For this review, use the dimensioned drawing (mm, ordinates from the lowest corner) and the shaded views. Give positions to 0.01 mm unless a question says otherwise; leave off trailing zeros. Order: outer loops, then holes, each group sorted by start corner. A loop starts at its lowest first (then second) coordinate and runs counter-clockwise, first axis right, second up. Notation, with made-up numbers: M 27.25,75 L 64.25,75 A15 cw 64.25,83 Z; hole C 74,-18.5 d7. An arc over 180 degrees is marked long. Answer as CSV lines item,"result". Start each with the question number.
1. We need section A-A, the plane y = 12. Give the boundary of the cut face in (x, z), and give its area (3 significant figures).
2. We need section C-C, the plane z = 7.25. Give the boundary of the cut face in (x, y).
3. Mouldability with a two-part tool opening along X and no side actions: class the marked faces 1, 2 and 3 as pulls with the +X half, pulls with the -X half, needs draft (parallel to the pull), parting line crosses it, or undercut.
4. For line 1 along Y through (x, z) = (12, 4.25); line 2 along Y through (x, z) = (8.5, 5.5); line 3 along Y through (x, z) = (22, 1.75), list the stretches that pass through material, from the lowest coordinate up.
5. Clearance check with flat-ended pins moving along their axes: P1, Ø3, axis at x = 8, z = 1.5, coming from the +Y side; P2, Ø3, axis at y = 8.5, z = 3.5, coming from the +X side. State where each tip first meets the part, or that it passes through.
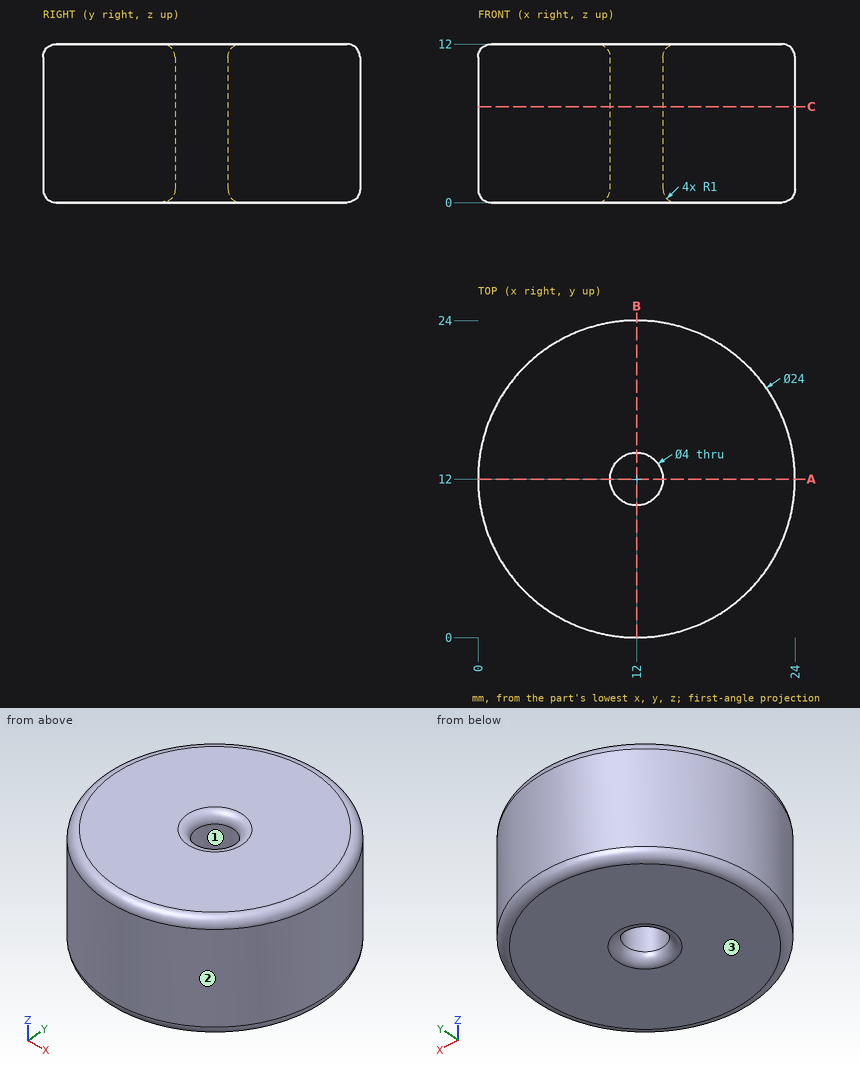
Result set:
1,outline,"M 0,1 A1 ccw 1,0 L 9,0 A1 ccw 10,1 L 10,11 A1 ccw 9,12 L 1,12 A1 ccw 0,11 Z; M 14,1 A1 ccw 15,0 L 23,0 A1 ccw 24,1 L 24,11 A1 ccw 23,12 L 15,12 A1 ccw 14,11 Z"
1,area,"238 mm2"
2,outline,"C 12,12 d24; hole C 12,12 d4"
3,face 1,"undercut"
3,face 2,"parting line crosses it"
3,face 3,"needs draft"
4,line 1,"0 to 10, 14 to 24"
4,line 2,"0.52 to 23.48"
4,line 3,"5.37 to 18.63"
5,P1,"y = 23.74"
5,P2,"x = 23.83"
